```python
from build123d import *

# Parameters (mm, degrees)
CUERPO_DEPTH                  = 28.5
CROQUIS_HUECO_ESP32_W         = 90.5
CROQUIS_HUECO_ESP32_H         = 57
HUECO_ESP32_DEPTH             = 18.4
CROQUIS_HUECO_PCB_W           = 90.5
CROQUIS_HUECO_PCB_H           = 52.5
HUECO_PCB_DEPTH               = 8.1
CROQUIS_LABIO_W               = 90.5
CROQUIS_LABIO_H               = 57
LABIO_LIP_DEPTH               = 2.4
CROQUIS_APOYOS_W              = 5
CROQUIS_APOYOS_H              = 5
APOYOS_PCB_DEPTH              = 4
CROQUIS_ALIVIOS_R             = 1
ALIVIOS_ESQUINAS_DEPTH        = 8.1
SALIDAS_USB_Y_PANEL_DEPTH     = 66.881977809
VENTILAS_LATERALES_DEPTH      = 66.881977809
VENTILAS_LATERALES_DEPTH_BACK = 66.881977809
REJILLA_PISO_DEPTH            = 2
CHAFLAN_BASE_SIZE             = 0.6


with BuildPart() as part:
    # Croquis_contorno → Cuerpo (new body)
    with BuildSketch(Plane(origin=(0, 0, 0), x_dir=(1, 0, 0), z_dir=(0, 1, 0))):
        with BuildLine():
            Line((-43.75, -28.75), (43.75, -28.75))
            ThreePointArc((43.75, -28.75), (46.578427125, -27.578427125), (47.75, -24.75))
            Line((47.75, -24.75), (47.75, 29.25))
            ThreePointArc((47.75, 29.25), (46.578427125, 32.078427125), (43.75, 33.25))
            Line((43.75, 33.25), (-43.75, 33.25))
            ThreePointArc((-43.75, 33.25), (-46.578427125, 32.078427125), (-47.75, 29.25))
            Line((-47.75, 29.25), (-47.75, -24.75))
            ThreePointArc((-47.75, -24.75), (-46.578427125, -27.578427125), (-43.75, -28.75))
        make_face()
    extrude(amount=CUERPO_DEPTH)

    # Croquis_hueco_ESP32 → Hueco_ESP32 (cut)
    with BuildSketch(Plane(origin=(0, 28.5, 0), x_dir=(1, 0, 0), z_dir=(0, 1, 0))):
        with Locations((0, 2.25)):
            Rectangle(CROQUIS_HUECO_ESP32_W, CROQUIS_HUECO_ESP32_H)
    extrude(amount=-HUECO_ESP32_DEPTH, mode=Mode.SUBTRACT)

    # Croquis_hueco_PCB → Hueco_PCB (cut)
    with BuildSketch(Plane(origin=(0, 10.1, 0), x_dir=(1, 0, 0), z_dir=(0, 1, 0))):
        Rectangle(CROQUIS_HUECO_PCB_W, CROQUIS_HUECO_PCB_H)
    extrude(amount=-HUECO_PCB_DEPTH, mode=Mode.SUBTRACT)

    # Croquis_labio → Labio_lip (add)
    with BuildSketch(Plane(origin=(0, 28.5, 0), x_dir=(1, 0, 0), z_dir=(0, 1, 0))):
        with BuildLine():
            Line((-43.75, -27.6), (43.75, -27.6))
            ThreePointArc((43.75, -27.6), (45.765254326, -26.765254326), (46.6, -24.75))
            Line((46.6, -24.75), (46.6, 29.25))
            ThreePointArc((46.6, 29.25), (45.765254326, 31.265254326), (43.75, 32.1))
            Line((43.75, 32.1), (-43.75, 32.1))
            ThreePointArc((-43.75, 32.1), (-45.765254326, 31.265254326), (-46.6, 29.25))
            Line((-46.6, 29.25), (-46.6, -24.75))
            ThreePointArc((-46.6, -24.75), (-45.765254326, -26.765254326), (-43.75, -27.6))
        make_face()
        with Locations((0, 2.25)):
            Rectangle(CROQUIS_LABIO_W, CROQUIS_LABIO_H, mode=Mode.SUBTRACT)
    extrude(amount=LABIO_LIP_DEPTH)

    # Croquis_apoyos → Apoyos_PCB (add)
    with BuildSketch(Plane(origin=(0, 2, 0), x_dir=(1, 0, 0), z_dir=(0, 1, 0))):
        with Locations((-42.75, -23.75)):
            Rectangle(CROQUIS_APOYOS_W, CROQUIS_APOYOS_H)
        with Locations((-42.75, 23.75)):
            Rectangle(CROQUIS_APOYOS_W, CROQUIS_APOYOS_H)
        with Locations((42.75, -23.75)):
            Rectangle(CROQUIS_APOYOS_W, CROQUIS_APOYOS_H)
        with Locations((42.75, 23.75)):
            Rectangle(CROQUIS_APOYOS_W, CROQUIS_APOYOS_H)
    extrude(amount=APOYOS_PCB_DEPTH)

    # Croquis_alivios → Alivios_esquinas (cut)
    with BuildSketch(Plane(origin=(0, 2, 0), x_dir=(1, 0, 0), z_dir=(0, 1, 0))):
        with Locations(Location((-45.25, -26.25, 0), (0, 0, 90))):
            Circle(CROQUIS_ALIVIOS_R)
        with Locations(Location((-45.25, 26.25, 0), (0, 0, 270))):
            Circle(CROQUIS_ALIVIOS_R)
        with Locations(Location((45.25, -26.25, 0), (0, 0, 90))):
            Circle(CROQUIS_ALIVIOS_R)
        with Locations(Location((45.25, 26.25, 0), (0, 0, 270))):
            Circle(CROQUIS_ALIVIOS_R)
    extrude(amount=ALIVIOS_ESQUINAS_DEPTH, mode=Mode.SUBTRACT)

    # Croquis_salidas → Salidas_USB_y_panel (cut, through all)
    with BuildSketch(Plane.XY):
        with BuildLine():
            Line((6.8, 23.1), (11.8, 23.1))
            ThreePointArc((11.8, 23.1), (15.8, 19.1), (11.8, 15.1))
            Line((11.8, 15.1), (6.8, 15.1))
            ThreePointArc((6.8, 15.1), (2.8, 19.1), (6.8, 23.1))
        make_face()
        with BuildLine():
            Line((-15.96, 15.6), (-10.96, 15.6))
            ThreePointArc((-10.96, 15.6), (-7.46, 12.1), (-10.96, 8.6))
            Line((-10.96, 8.6), (-15.96, 8.6))
            ThreePointArc((-15.96, 8.6), (-19.46, 12.1), (-15.96, 15.6))
        make_face()
    extrude(amount=-SALIDAS_USB_Y_PANEL_DEPTH, mode=Mode.SUBTRACT)

    # Croquis_ventilas → Ventilas_laterales (cut, two sides: drawn at the far end of the back side and taken through both)
    with BuildSketch(Plane(origin=(0, 0, 0), x_dir=(0, 0, -1), z_dir=(1, 0, 0)).offset(-VENTILAS_LATERALES_DEPTH_BACK)):
        with BuildLine():
            Line((-18.609650045, 13.003805922), (-7.295941546, 24.317514421))
            ThreePointArc((-7.295941546, 24.317514421), (-5.174621202, 24.317514421), (-5.174621202, 22.196194078))
            Line((-5.174621202, 22.196194078), (-16.488329701, 10.882485579))
            ThreePointArc((-16.488329701, 10.882485579), (-18.609650045, 10.882485579), (-18.609650045, 13.003805922))
        make_face()
        with BuildLine():
            Line((-11.538582233, 13.003805922), (-0.224873734, 24.317514421))
            ThreePointArc((-0.224873734, 24.317514421), (1.896446609, 24.317514421), (1.896446609, 22.196194078))
            Line((1.896446609, 22.196194078), (-9.41726189, 10.882485579))
            ThreePointArc((-9.41726189, 10.882485579), (-11.538582233, 10.882485579), (-11.538582233, 13.003805922))
        make_face()
        with BuildLine():
            Line((-4.467514421, 13.003805922), (6.846194078, 24.317514421))
            ThreePointArc((6.846194078, 24.317514421), (8.967514421, 24.317514421), (8.967514421, 22.196194078))
            Line((8.967514421, 22.196194078), (-2.346194078, 10.882485579))
            ThreePointArc((-2.346194078, 10.882485579), (-4.467514421, 10.882485579), (-4.467514421, 13.003805922))
        make_face()
        with BuildLine():
            Line((2.603553391, 13.003805922), (13.91726189, 24.317514421))
            ThreePointArc((13.91726189, 24.317514421), (16.038582233, 24.317514421), (16.038582233, 22.196194078))
            Line((16.038582233, 22.196194078), (4.724873734, 10.882485579))
            ThreePointArc((4.724873734, 10.882485579), (2.603553391, 10.882485579), (2.603553391, 13.003805922))
        make_face()
        with BuildLine():
            Line((9.674621202, 13.003805922), (20.988329701, 24.317514421))
            ThreePointArc((20.988329701, 24.317514421), (23.109650045, 24.317514421), (23.109650045, 22.196194078))
            Line((23.109650045, 22.196194078), (11.795941546, 10.882485579))
            ThreePointArc((11.795941546, 10.882485579), (9.674621202, 10.882485579), (9.674621202, 13.003805922))
        make_face()
    extrude(amount=VENTILAS_LATERALES_DEPTH + VENTILAS_LATERALES_DEPTH_BACK, mode=Mode.SUBTRACT)

    # Croquis_rejilla_piso → Rejilla_piso (cut)
    with BuildSketch(Plane(origin=(0, 0, 0), x_dir=(1, 0, 0), z_dir=(0, 1, 0))):
        with BuildLine():
            Line((-36.769552622, -11.185028843), (-7.778174593, 17.806349186))
            ThreePointArc((-7.778174593, 17.806349186), (-5.656854249, 17.806349186), (-5.656854249, 15.685028843))
            Line((-5.656854249, 15.685028843), (-34.648232278, -13.306349186))
            ThreePointArc((-34.648232278, -13.306349186), (-36.769552622, -13.306349186), (-36.769552622, -11.185028843))
        make_face()
        with BuildLine():
            Line((-29.69848481, -11.185028843), (-1.060660172, 17.452795796))
            ThreePointArc((-1.060660172, 17.452795796), (1.060660172, 17.452795796), (1.060660172, 15.331475452))
            Line((1.060660172, 15.331475452), (-27.577164466, -13.306349186))
            ThreePointArc((-27.577164466, -13.306349186), (-29.69848481, -13.306349186), (-29.69848481, -11.185028843))
        make_face()
        with BuildLine():
            Line((-22.273863607, -11.185028843), (6.363961031, 17.452795796))
            ThreePointArc((6.363961031, 17.452795796), (8.485281374, 17.452795796), (8.485281374, 15.331475452))
            Line((8.485281374, 15.331475452), (-20.152543264, -13.306349186))
            ThreePointArc((-20.152543264, -13.306349186), (-22.273863607, -13.306349186), (-22.273863607, -11.185028843))
        make_face()
        with BuildLine():
            Line((-15.379572491, -11.185028843), (13.258252147, 17.452795796))
            ThreePointArc((13.258252147, 17.452795796), (15.379572491, 17.452795796), (15.379572491, 15.331475452))
            Line((15.379572491, 15.331475452), (-13.258252147, -13.306349186))
            ThreePointArc((-13.258252147, -13.306349186), (-15.379572491, -13.306349186), (-15.379572491, -11.185028843))
        make_face()
        with BuildLine():
            Line((-7.954951288, -11.185028843), (20.68287335, 17.452795796))
            ThreePointArc((20.68287335, 17.452795796), (22.804193693, 17.452795796), (22.804193693, 15.331475452))
            Line((22.804193693, 15.331475452), (-5.833630945, -13.306349186))
            ThreePointArc((-5.833630945, -13.306349186), (-7.954951288, -13.306349186), (-7.954951288, -11.185028843))
        make_face()
        with BuildLine():
            Line((-1.060660172, -11.185028843), (27.577164466, 17.452795796))
            ThreePointArc((27.577164466, 17.452795796), (29.69848481, 17.452795796), (29.69848481, 15.331475452))
            Line((29.69848481, 15.331475452), (1.060660172, -13.306349186))
            ThreePointArc((1.060660172, -13.306349186), (-1.060660172, -13.306349186), (-1.060660172, -11.185028843))
        make_face()
        with BuildLine():
            Line((5.303300859, -11.185028843), (34.471455583, 17.983125881))
            ThreePointArc((34.471455583, 17.983125881), (36.592775926, 17.983125881), (36.592775926, 15.861805538))
            Line((36.592775926, 15.861805538), (7.424621202, -13.306349186))
            ThreePointArc((7.424621202, -13.306349186), (5.303300859, -13.306349186), (5.303300859, -11.185028843))
        make_face()
    extrude(amount=REJILLA_PISO_DEPTH, mode=Mode.SUBTRACT)

    # Chaflan_base
    chaflan_base_edges = [part.edges().sort_by_distance(p)[0] for p in [
        (47.75, 0, -2.25),
        (46.578427125, 0, 27.578427125),
        (0, 0, 28.75),
        (-46.578427125, 0, 27.578427125),
        (-47.75, 0, -2.25),
        (-46.578427125, 0, -32.078427125),
        (0, 0, -33.25),
        (46.578427125, 0, -32.078427125),
    ]]
    chamfer(chaflan_base_edges, length=CHAFLAN_BASE_SIZE)


solid = part.part
```
Can you work these out from the model? Positions are in its coordinate system, mm. A direction names the side the tool comes from. Coordinates: 2 decimals unless noted, no trailing zeros. Order: outer loops, then holes, each group sorted by start corner. A loop starts at its lowest first (then second) coordinate and runs counter-clockwise, first axis right, second up.
1. I need wall thicknesses on line 1 (Z direction, x = -10.5, y = 18); line 2 (Z direction, x = -5.5, y = 29.5); line 3 (Z direction, x = -45, y = 4). Which ranges of each line are inside material? Lowest first, please.
2. If we section it at A-A (x = 18): Please give me the cut outline in (y, z).
3. Thinking about a two-plate mould opening in Z: for faces 1 (the face through (0, 30.9, -31)), 2 (the face through (-45, 2, -26)), which applies, +Z half, -Z half, draft (parallel to the pull), parting line (faces both ways), or undercut?
4. For faces 3 (the face through (45, 2, 26)), 4 (the face through (-40.25, 4, 24)), 5 (the face through (-15.58, 0.986, -2.933)), 6 (the face through (-46.52, 18.58, 5.96)), which set-ups out of +Z, -Z, +X, -X, +Y, -Y let a thin tool reach every point of the face, with its end or its side?
5. I'm going to push flat-ended pins straight in: pin 1 (0.7 mm diameter, centred on x = 7, y = 29.5, fed in from -Z); pin 2 (4 mm diameter, centred on x = -42, z = -23, fed in from +Y); pin 3 (12 mm diameter, centred on x = -35.5, z = 13.5, fed in from +Y). Where does each tip first touch, or does it pass through?
6. If we section it at B-B (z = 3.5): Give the number of separate pieces and of enclosed holes in the cut face, then the cut area to 3 significant figures.
Entries:
1. line 1: z = -33.25 to -30.75, 26.25 to 28.75
1. line 2: z = -32.1 to -30.75, 26.25 to 27.6
1. line 3: z = -33.05 to -27.22, -25.28 to -21.25, 21.25 to 25.28, 27.22 to 28.55
2. outline: (0, -32.65) - (0.6, -33.25) - (28.5, -33.25) - (28.5, -32.1) - (30.9, -32.1) - (30.9, -30.75) - (10.1, -30.75) - (10.1, -26.25) - (2, -26.25) - (2, -14.77) - (0, -14.77) - close; (0, -10.53) - (2, -10.53) - (2, -7.88) - (0, -7.88) - close; (0, -3.63) - (2, -3.63) - (2, -1.51) - (0, -1.51) - close; (0, 2.73) - (2, 2.73) - (2, 26.25) - (30.9, 26.25) - (30.9, 27.6) - (28.5, 27.6) - (28.5, 28.75) - (0.6, 28.75) - (0, 28.15) - close
3. face 1: draft
3. face 2: undercut
4. face 3: none
4. face 4: +Y
4. face 5: +Y, -Y
4. face 6: +X, -X
5. pin 1: stops at z = -32.1
5. pin 2: stops at y = 6
5. pin 3: stops at y = 2
6. separate pieces: 12
6. enclosed holes: 0
6. area: 231 mm2
